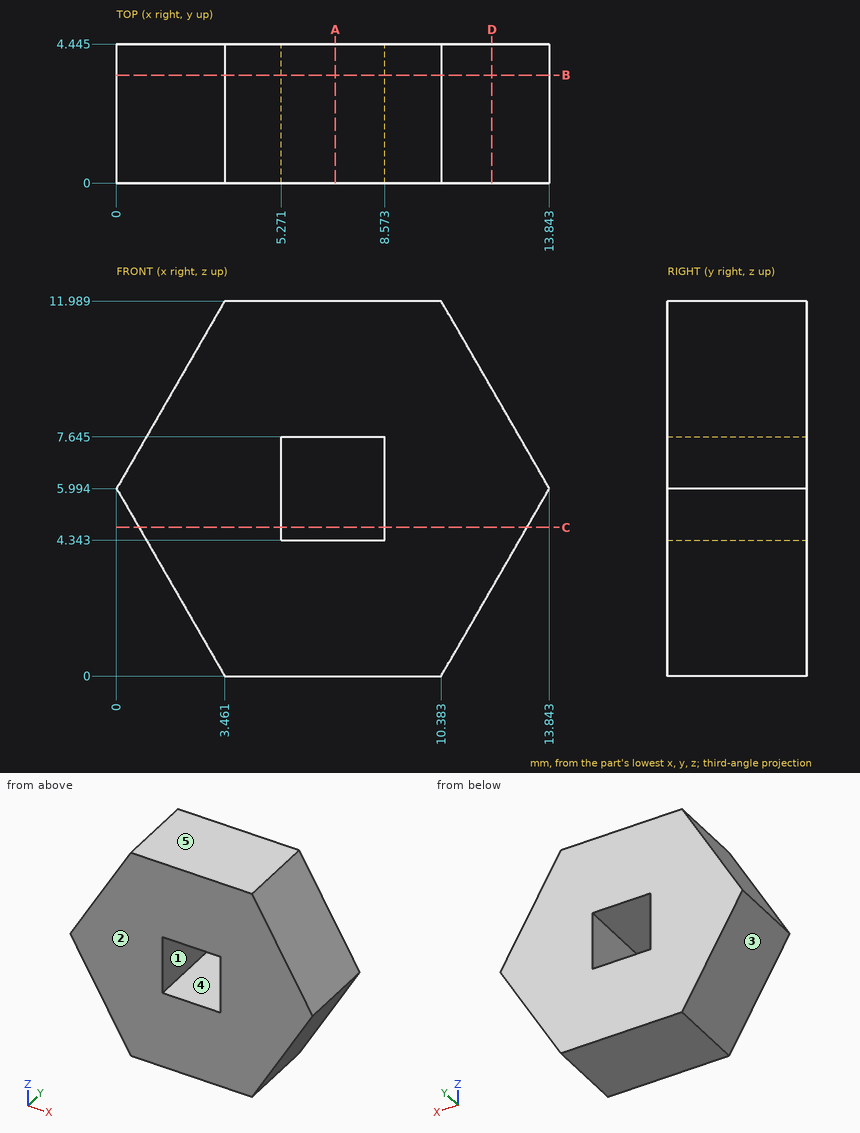
Could you check a few things on this drawing? It's one solid part, dimensions in mm from its lowest x, y, z. A direction names the side the tool comes from. Give positions to 0.01 mm unless a question says otherwise; leave off trailing zeros. Loops run counter-clockwise (first coordinate to the right, second up) from the corner with the lowest first, then second, coordinate; pieces in that order, holes last. Notation, with made-up numbers: M -19.5,77.25 L 10.5,77.25 A18 cw 10.5,87.25 Z; hole C 5,67 d11. An arc over 180 degrees is marked long. Return JSON: item names as keys, results as strings.
Item 1: Imagine slicing it at C-C on z = 4.75. List the corners of the cut face in (x, y) for me (1 decimal).
A:
{"outline": "M 0.7,0 L 5.3,0 L 5.3,4.4 L 0.7,4.4 Z; M 8.6,0 L 13.1,0 L 13.1,4.4 L 8.6,4.4 Z"}
Item 2: Imagine slicing it at A-A on x = 7. List the corners of the cut face in (y, z) for me (1 decimal).
A:
{"outline": "M 0,0 L 4.4,0 L 4.4,4.3 L 0,4.3 Z; M 0,7.6 L 4.4,7.6 L 4.4,12 L 0,12 Z"}
Item 3: I'm going to push a flat-ended pin straight in: pin 1 Ø6 at (x, z) = (8.5, 4.5) entering from -Y. Where does the tip first touch, or does it pass through?
A:
{"pin 1": "stops at y = 0"}
Item 4: On a 3-axis mill with a long thin cutter (end or side, diameter ignored), from which of +Z, -Z, +X, -X, +Y, -Y can I reach the whole of each face in a straight line? I mean the marked faces 1 and 2. Say none if no direction works.
A:
{"face 1": "+Y, -Y", "face 2": "+Z, -Z, +X, -X, -Y"}
Item 5: Imagine slicing it at D-D on x = 12. List the corners of the cut face in (y, z) for me (1 decimal), then the cut area to 3 significant figures.
A:
{"outline": "M 0,2.8 L 4.4,2.8 L 4.4,9.2 L 0,9.2 Z", "area": "28.4 mm^2"}
Item 6: Imagine slicing it at B-B on y = 3.45. List the corners of the cut face in (x, z) for me (1 decimal), then the cut area to 3 significant figures.
A:
{"outline": "M 0,6 L 3.5,0 L 10.4,0 L 13.8,6 L 10.4,12 L 3.5,12 Z; hole M 5.3,4.3 L 8.6,4.3 L 8.6,7.6 L 5.3,7.6 Z", "area": "114 mm^2"}
Item 7: Please list where these lines run through material, in increasing order: line 1 (Z direction, x = 7.5, y = 1.5) (1 decimal); line 2 (X direction, y = 3.5, z = 6.25) (1 decimal); line 3 (X direction, y = 2.6, z = 5) (1 decimal).
A:
{"line 1": "z = 0 to 4.3, 7.6 to 12", "line 2": "x = 0.1 to 5.3, 8.6 to 13.7", "line 3": "x = 0.6 to 5.3, 8.6 to 13.3"}
Item 8: Thinking about a two-plate mould opening in Z: for the marked faces 3, 4 and 5, which applies, released by +Z, released by -Z, zero draft, split by the parting line, or undercut?
A:
{"face 3": "released by -Z", "face 4": "undercut", "face 5": "released by +Z"}
